```python
from build123d import *

# Parameters (mm, degrees)
SKETCH1_R                                  = 82.5
SKETCH1_R_2                                = 55
BOSS_EXTRUDE1_DEPTH                        = 62
SKETCH6_R                                  = 61
BOSS_EXTRUDE4_DEPTH                        = 10
SKETCH8_R                                  = 40.25
CUT_EXTRUDE4_DEPTH                         = 10
SKETCH9_R                                  = 2.7
CUT_EXTRUDE5_DEPTH                         = 30
CIRPATTERN6_COUNT                          = 10
SKETCH10_R                                 = 4.66
CUT_EXTRUDE6_DEPTH                         = 7.62
CIRPATTERN7_COUNT                          = 6
SKETCH12_W                                 = 20
SKETCH12_H                                 = 41
CUT_EXTRUDE7_DEPTH                         = 11.3
SKETCH13_R                                 = 4.66
CUT_EXTRUDE8_DEPTH                         = 7.62
MIRROR2_AT_THE_SECOND_PLANE_COPY_1_SKETC_R = 4.66
MIRROR2_AT_THE_SECOND_PLANE_COPY_1_DEPTH   = 7.62


with BuildPart() as part:
    # Sketch1 → Boss-Extrude1 (new body)
    with BuildSketch(Plane(origin=(0, 0, 0), x_dir=(1, 0, 0), z_dir=(0, 1, 0))):
        with Locations(Location((0, 0, 0), (0, 0, 270))):
            Circle(SKETCH1_R)
        with Locations(Location((0, 0, 0), (0, 0, 270))):
            Circle(SKETCH1_R_2, mode=Mode.SUBTRACT)
    extrude(amount=BOSS_EXTRUDE1_DEPTH)

    # Sketch6 → Boss-Extrude4 (add)
    with BuildSketch(Plane(origin=(0, 62, 0), x_dir=(1, 0, 0), z_dir=(0, 1, 0))):
        with Locations(Location((0, 0, 0), (0, 0, 270))):
            Circle(SKETCH6_R)
    extrude(amount=BOSS_EXTRUDE4_DEPTH)

    # Sketch8 → Cut-Extrude4 (cut)
    with BuildSketch(Plane(origin=(0, 72, 0), x_dir=(1, 0, 0), z_dir=(0, 1, 0))):
        with Locations(Location((0, 0, 0), (0, 0, 270))):
            Circle(SKETCH8_R)
    extrude(amount=-CUT_EXTRUDE4_DEPTH, mode=Mode.SUBTRACT)

    # Sketch9 → Cut-Extrude5 (cut)
    with BuildSketch(Plane(origin=(0, 72, 0), x_dir=(1, 0, 0), z_dir=(0, 1, 0))):
        with Locations(Location((0, 48.5, 0), (0, 0, 270))):
            Circle(SKETCH9_R)
    cut_extrude5 = extrude(amount=-CUT_EXTRUDE5_DEPTH, mode=Mode.SUBTRACT)

    # CirPattern6: Cut-Extrude5 ×10 about axis
    cirpattern6_axis = Axis((0, 0, 0), (0, 1, 0))
    for i in range(1, CIRPATTERN6_COUNT):
        add(cut_extrude5.rotate(cirpattern6_axis, i * 360 / CIRPATTERN6_COUNT), mode=Mode.SUBTRACT)

    # Sketch10 → Cut-Extrude6 (cut)
    with BuildSketch(Plane.XZ):
        with Locations(Location((0, 69.5, 0), (0, 0, 270))):
            Circle(SKETCH10_R)
    cut_extrude6 = extrude(amount=-CUT_EXTRUDE6_DEPTH, mode=Mode.SUBTRACT)

    # CirPattern7: Cut-Extrude6 ×6 about axis
    cirpattern7_axis = Axis((0, 0, 0), (0, 1, 0))
    for i in range(1, CIRPATTERN7_COUNT):
        add(cut_extrude6.rotate(cirpattern7_axis, i * 360 / CIRPATTERN7_COUNT), mode=Mode.SUBTRACT)

    # Sketch12 → Cut-Extrude7 (cut)
    with BuildSketch(Plane.XZ):
        with Locations((61.036751464, 0)):
            Rectangle(SKETCH12_W, SKETCH12_H)
    cut_extrude7 = extrude(amount=-CUT_EXTRUDE7_DEPTH, mode=Mode.SUBTRACT)

    # Mirror1: Cut-Extrude7 across plane
    add(cut_extrude7.mirror(Plane(origin=(0, 0, 0), x_dir=(0, 0, 1), z_dir=(1, 0, 0))), mode=Mode.SUBTRACT)

    # Sketch13 → Cut-Extrude8 (cut)
    with BuildSketch(Plane.XZ.offset(-11.3)):
        with Locations(Location((63, 10.5, 0), (0, 0, 270))):
            Circle(SKETCH13_R)
    cut_extrude8 = extrude(amount=-CUT_EXTRUDE8_DEPTH, mode=Mode.SUBTRACT)

    # Mirror2: Cut-Extrude8 across plane
    add(cut_extrude8.mirror(Plane(origin=(0, 0, 0), x_dir=(0, 0, 1), z_dir=(1, 0, 0))), mode=Mode.SUBTRACT)

    # Mirror2 at the second plane: Cut-Extrude8 across plane
    add(cut_extrude8.mirror(Plane.XY), mode=Mode.SUBTRACT)

    # Mirror2 at the second plane copy 1 sketc → Mirror2 at the second plane copy 1 (cut)
    with BuildSketch(Plane(origin=(0, 11.3, 0), x_dir=(-1, 0, 0), z_dir=(0, -1, 0))):
        with Locations(Location((63, 10.5, 0), (0, 0, 270))):
            Circle(MIRROR2_AT_THE_SECOND_PLANE_COPY_1_SKETC_R)
    extrude(amount=-MIRROR2_AT_THE_SECOND_PLANE_COPY_1_DEPTH, mode=Mode.SUBTRACT)


solid = part.part
```
Design review of the part built by this model. Coordinates are the model's own, in mm. A direction names the side the tool comes from. Give positions to 0.01 mm unless a question says otherwise; leave off trailing zeros. Order: outer loops, then holes, each group sorted by start corner. A loop starts at its lowest first (then second) coordinate and runs counter-clockwise, first axis right, second up. Notation, with made-up numbers: (46.5, 75.5) - (61.5, 75.5) arc R28 cw to (61.5, 96.5) - close; hole circle Ø2 at (-17, 21). An arc over 180 degrees is marked (long way). Use a Markdown table: item, result. Add a question column.
(1) Wall thickness on probe 1 along X at (y, z) = (60, -45); probe 2 along Z at (x, y) = (39.5, 8.5); probe 3 along Z at (x, y) = (-13, 61): over which ranges is each line inside the solid? List them lowest first. Write a range as [from, to].
(2) Add section A-A on z = 0. Give the boundary of the cut face in (x, y).
(3) Clearance check with flat-ended pins moving along their axes: P1, Ø4.5, axis at x = 60, z = 35, coming from the -Y side; P2, Ø12, axis at x = 63, z = 10.5, coming from the -Y side; P3, Ø8, axis at x = 25.5, y = 39.5, coming from the +Z side; P4, Ø8, axis at x = -54.5, z = 49.5, coming from the -Y side. State where each tip first meets the part, or that it passes through.
(4) Add section C-C on y = 25. Give the boundary of the cut face in (x, z).
(5) Mouldability with a two-part tool opening along X and no side actions: class faces 3 (the face through (-60, 7.62, 35)), 4 (the face through (-36.3, 62, -49.3)), 5 (the face through (-59.55, 66.93, -13.22)) as +X half, -X half, draft (parallel to the pull), parting line (faces both ways), or undercut.
(6) Add section B-B on x = 0. Give the number of separate pieces and of enclosed holes in the cut face, then the cut area to 3 significant figures.
(7) Add section D-D on z = 48.5. Give the boundary of the cut face in (x, y).
(8) Machinability: for faces 1 (the face through (0.811, 67.07, -45.925)), 2 (the face through (-0.205, 3.757, -74.155)), which of the approach directions +Z, -Z, +X, -X, +Y, -Y give a long, thin tool a straight path to every point of the face, cutting with its end or side? Answer none if there is none.
Report:
| question | item | result |
|---|---|---|
| 1 | probe 1 | x = [-69.15, -31.62], [31.62, 69.15] |
| 1 | probe 2 | z = [-72.43, -38.27], [38.27, 72.43] |
| 1 | probe 3 | z = [-81.47, -53.44], [53.44, 81.47] |
| 2 | outline | (-82.5, 0) - (-71.04, 0) - (-71.04, 11.3) - (-55, 11.3) - (-55, 62) - (-40.25, 62) - (-40.25, 72) - (-61, 72) - (-61, 62) - (-82.5, 62) - close; (40.25, 62) - (55, 62) - (55, 11.3) - (71.04, 11.3) - (71.04, 0) - (82.5, 0) - (82.5, 62) - (61, 62) - (61, 72) - (40.25, 72) - close |
| 3 | P1 | stops at y = 7.62 |
| 3 | P2 | stops at y = 11.3 |
| 3 | P3 | stops at z = 79.65 |
| 3 | P4 | stops at y = 0 |
| 4 | outline | circle Ø165 at (0, 0); hole circle Ø110 at (0, 0) |
| 5 | face 3 | undercut |
| 5 | face 4 | draft |
| 5 | face 5 | parting line |
| 6 | separate pieces | 4 |
| 6 | enclosed holes | 0 |
| 6 | area | 3,570 mm² |
| 7 | outline | (-66.74, 0) - (-25.94, 0) - (-25.94, 62) - (-2.7, 62) - (-2.7, 72) - (-37, 72) - (-37, 62) - (-66.74, 62) - close; (2.7, 62) - (25.94, 62) - (25.94, 0) - (66.74, 0) - (66.74, 62) - (37, 62) - (37, 72) - (2.7, 72) - close |
| 8 | face 1 | +Y, -Y |
| 8 | face 2 | -Y |
